from build123d import *

# Parameters (mm, degrees)
F0_R     = 19.05
F1_DEPTH = 25.4
F2_DEPTH = 99.822
F4_DEPTH = 250.19
F5_DEPTH = 250.19
F6_W     = 161.29
F6_H     = 62.738
F6_H_2   = 49.2019202976
F7_DEPTH = 171.704


# Not quite as in the source:
# - a feature names something its author has since deleted; it is built from what else it names


with BuildPart() as f1:
    # F0 (on Front) → F1 (new body, symmetric)
    with BuildSketch(Plane.XZ):
        with BuildLine():
            ThreePointArc((0, 38.1), (11.1592316368, 11.1592316368), (38.1, 0))
            Line((38.1, 0), (215.9, 0))
            ThreePointArc((215.9, 0), (242.8407683632, 11.1592316368), (254, 38.1))
            Line((254, 38.1), (254, 266.7))
            ThreePointArc((254, 266.7), (242.8407683632, 293.6407683632), (215.9, 304.8))
            Line((215.9, 304.8), (38.1, 304.8))
            ThreePointArc((38.1, 304.8), (11.1592316368, 293.6407683632), (0, 266.7))
            Line((0, 266.7), (0, 38.1))
        make_face()
        with BuildLine():
            ThreePointArc((57.0266099035, 35.9352973504), (37.3773915988, 19.0637099965), (19.0637495923, 37.376349246))
            ThreePointArc((19.0637495923, 37.376349246), (37.7381093173, 57.1465622918), (57.15, 38.1))
            ThreePointArc((57.15, 38.1), (57.1191274598, 37.0158917631), (57.0266099035, 35.9352973504))
        make_face(mode=Mode.SUBTRACT)
        Polygon((248.4933634432, 89.814005202), (189.582883289, 30.9035250478), (12.671837704, 207.8145706329), (71.5823178582, 266.7250507871), align=None, mode=Mode.SUBTRACT)
        with Locations((215.9, 266.7)):
            Circle(F0_R, mode=Mode.SUBTRACT)
        Polygon((12.671837704, 207.8145706329), (189.582883289, 30.9035250478), (248.4933634432, 89.814005202), (71.5823178582, 266.7250507871), align=None)
    extrude(amount=F1_DEPTH, both=True)

    # F0 (on Front) → F2 (join)
    with BuildSketch(Plane.XZ):
        Polygon((12.671837704, 207.8145706329), (189.582883289, 30.9035250478), (248.4933634432, 89.814005202), (71.5823178582, 266.7250507871), align=None)
    extrude(amount=F2_DEPTH)

    # F3 (on face) → F4 (join)
    with BuildSketch(Plane(origin=(79.3396791206, 0, -79.3396791206), x_dir=(0, 1, 0), z_dir=(0.7071067812, 0, -0.7071067812))):
        with BuildLine():
            ThreePointArc((-99.822, 168.3534344944), (-129.032, 197.5634344944), (-99.822, 226.7734344944))
            Line((-99.822, 226.7734344944), (-99.822, 239.2194344944))
            ThreePointArc((-99.822, 239.2194344944), (-141.478, 197.5634344944), (-99.822, 155.9074344944))
            Line((-99.822, 155.9074344944), (-99.822, 168.3534344944))
        make_face()
    extrude(amount=-F4_DEPTH)

    # F3 (on face) → F5 (cut)
    with BuildSketch(Plane(origin=(79.3396791206, 0, -79.3396791206), x_dir=(0, 1, 0), z_dir=(0.7071067812, 0, -0.7071067812))):
        with BuildLine():
            ThreePointArc((-99.822, 168.3534344944), (-79.1674109215, 176.908845416), (-70.612, 197.5634344944))
            ThreePointArc((-70.612, 197.5634344944), (-79.1674109215, 218.2180235729), (-99.822, 226.7734344944))
            Line((-99.822, 226.7734344944), (-99.822, 168.3534344944))
        make_face()
    extrude(amount=-F5_DEPTH, mode=Mode.SUBTRACT)

    # F6 (on face) → F7 (cut)
    with BuildSketch(Plane(origin=(110.2432041684, 0, 110.2432041684), x_dir=(0.7071067812, 0, -0.7071067812), z_dir=(-0.7071067812, 0, -0.7071067812))):
        with Locations((-12.8917497533, 68.453)):
            Rectangle(F6_W, F6_H)
        with Locations((-12.8917497533, 124.4229601488)):
            Rectangle(F6_W, F6_H_2)
    extrude(amount=-F7_DEPTH, mode=Mode.SUBTRACT)


solid = f1.part
Could you check a few things on this model? Use its own coordinates, in mm. A direction names the side the tool comes from. Round coordinates to 2 decimals unless told otherwise and drop trailing zeros. Write each loop counter-clockwise with the first axis right and the second up, starting at its lowest first coordinate (ties: lowest second). Pieces come first, ordered by that corner, then holes. Notation, with made-up numbers: (10.25, 77.5) - (68.25, 77.5) arc R20 ccw to (68.25, 91.5) - close; hole circle Ø8 at (70.25, -17.75). An arc over 180 degrees is marked (long way). Use a Markdown table: item, result.
Q1. I want a section at B-B (z = 275). List the corners of the cut face in (x, y) for me.
Output values:
| item | result |
|---|---|
| outline | (0.92, -25.4) - (198.75, -25.4) - (198.75, 25.4) - (0.92, 25.4) - close; (233.05, -25.4) - (253.08, -25.4) - (253.08, 25.4) - (233.05, 25.4) - close |
Q2. Thinking about a two-plate mould opening in Z: for faces 5 (the flat face through (153, -25.4, 188)), 6 (the cylindrical face through (234.07, 0.36, 272.42)), 7 (the flat face through (128, 0, 304.8)), which applies, released by +Z, released by -Z, zero draft, split by the parting line, or undercut?
Output values:
| item | result |
|---|---|
| face 5 | zero draft |
| face 6 | undercut |
| face 7 | released by +Z |
Q3. For pin 1 (6 mm diameter, centred on x = 61, y = -48.5, fed in from +Z); pin 2 (4 mm diameter, centred on x = 199, y = -70.5, fed in from -Z); pin 3 (1 mm diameter, centred on y = -81.5, z = 98, fed in from -X), each with a flat end and sliding along its axis, tell me the tip position at first contact or that it passes through.
Output values:
| item | result |
|---|---|
| pin 1 | z = 259.14 |
| pin 2 | z = 38.32 |
| pin 3 | x = 212.8 |
Q4. Please list where these lines run through material, in increasing order: L1, parallel to Z at x = 215.9, y = 2; L2, parallel to X at y = 7, z = 38; L3, parallel to Y at x = 46, z = 171.5.
Output values:
| item | result |
|---|---|
| L1 | 0 to 247.65, 285.75 to 304.8 |
| L2 | 0 to 19.05, 57.15 to 254 |
| L3 | -25.4 to 25.4 |
Q5. I want a section at A-A (y = -114). List the corners of the cut face in (x, z) for me.
Output values:
| item | result |
|---|---|
| outline | (14.43, 209.57) - (45.86, 178.14) - (55.5, 187.78) - (24.07, 219.21) - close; (60.19, 255.33) - (91.62, 223.9) - (101.25, 233.54) - (69.82, 264.97) - close; (159.91, 64.09) - (191.34, 32.66) - (200.98, 42.3) - (169.55, 73.73) - close; (205.67, 109.85) - (237.1, 78.42) - (246.73, 88.06) - (215.3, 119.49) - close |
Q6. For faces 1 (the flat face through (49.09, -71.35, 244.23)), 2 (the flat face through (129, -37.084, 149)), 3 (the flat face through (226, -71.35, 67.32)), 4 (the flat face through (161.28, -29.01, 177.03)), which set-ups out of +Z, -Z, +X, -X, +Y, -Y let a thin tool reach every point of the face, with its end or its side?
Output values:
| item | result |
|---|---|
| face 1 | +Z, -X, -Y |
| face 2 | -Y |
| face 3 | -Z, +X, -Y |
| face 4 | +Z, +X, -Y |
